The model under review builds one solid part; all positions refer to its coordinate system, in mm. Coordinates: 2 decimals unless noted, no trailing zeros. Loops run counter-clockwise (first coordinate to the right, second up) from the corner with the lowest first, then second, coordinate; pieces in that order, holes last. Notation, with made-up numbers: (79, -37) - (94, -37) arc R24 ccw to (94, -16) - close; hole circle Ø6 at (-11.75, -4.5). An arc over 180 degrees is marked (long way). One line per item, written item: value. Start each with the question number.
1. We need section D-D, the plane x = 5.85. Give the boundary of the cut face in (y, z), then the cut area to 3 significant figures.
2. To check wall thickness, follow line 1 (Y direction, x = 6, z = 1.2); line 2 (X direction, y = 13.5, z = 0.2); line 3 (Y direction, x = 31, z = 0.55). State the ranges of each line that lie inside material, in increasing order.
3. We need section B-B, the plane x = 21.35. Give the boundary of the cut face in (y, z), then the cut area to 3 significant figures.
4. We need section A-A, the plane y = 43.4. Give the boundary of the cut face in (x, z), then the cut area to 3 significant figures.
5. We need section C-C, the plane z = 1.9. Give the boundary of the cut face in (x, y).
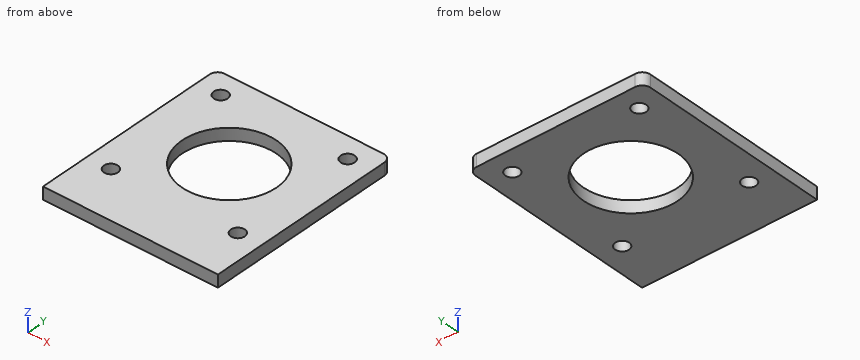
Autodesk Fusion 360 part; units mm, degrees
sketch "Sketch1" plane through (0, 0, 0) normal (0, 0, 1) x (1, 0, 0)
  line L0 (0, 0) -> (42.7, 0)
  line L1 (42.7, 0) -> (42.7, 49)
  line L2 (42.7, 49) -> (0, 49)
  line L3 (0, 49) -> (0, 0)
  circle A0 centre (21.35, 27.9) radius 11.5
  circle A1 centre (5.85, 43.4) radius 1.7
  line L4 (21.35, 49) -> (21.35, 0) construction
  circle A2 centre (5.85, 12.4) radius 1.7
  circle A3 centre (36.85, 43.4) radius 1.7
  circle A4 centre (36.85, 12.4) radius 1.7
  dimension "d1" = 49
  dimension "d2" = 42.7
  dimension "d3" = 9.6
  dimension "d4" = 15.5
  dimension "d5" = 15.5
  dimension "d6" = 3.4
  dimension "d9" = 31
  dimension "d10" = 31
  dimension "d11" = 23
extrude "Extrude1" add sketch "Sketch1" along normal blind 3
fillet "Fillet1" radius 2 2 edges at (0, 49, 1.5) (42.7, 49, 1.5)
Findings below:
1. outline: (0, 0) - (10.7, 0) - (10.7, 3) - (0, 3) - close; (14.1, 0) - (41.7, 0) - (41.7, 3) - (14.1, 3) - close; (45.1, 0) - (49, 0) - (49, 3) - (45.1, 3) - close
1. area: 127 mm2
2. line 1: 0 to 10.71, 14.09 to 41.71, 45.09 to 49
2. line 2: 0 to 4.55, 7.15 to 35.55, 38.15 to 42.7
2. line 3: 0 to 21.64, 34.16 to 49
3. outline: (0, 0) - (16.4, 0) - (16.4, 3) - (0, 3) - close; (39.4, 0) - (49, 0) - (49, 3) - (39.4, 3) - close
3. area: 78.0 mm2
4. outline: (0, 0) - (4.15, 0) - (4.15, 3) - (0, 3) - close; (7.55, 0) - (35.15, 0) - (35.15, 3) - (7.55, 3) - close; (38.55, 0) - (42.7, 0) - (42.7, 3) - (38.55, 3) - close
4. area: 108 mm2
5. outline: (0, 0) - (42.7, 0) - (42.7, 47) arc R2 ccw to (40.7, 49) - (2, 49) arc R2 ccw to (0, 47) - close; hole circle Ø3.4 at (5.85, 12.4); hole circle Ø3.4 at (5.85, 43.4); hole circle Ø23 at (21.35, 27.9); hole circle Ø3.4 at (36.85, 12.4); hole circle Ø3.4 at (36.85, 43.4)
